Source: three-view drawing plus pictorial views. Frame: mm from the lowest corner of the part. Give positions to 0.01 mm unless a question says otherwise; leave off trailing zeros. Loops run counter-clockwise (first coordinate to the right, second up) from the corner with the lowest first, then second, coordinate; pieces in that order, holes last. Notation, with made-up numbers: (5.25, 73.5) -> (33.25, 73.5) arc R9 ccw to (33.25, 80.5) -> close; hole circle Ø6 at (51, 57). An arc over 180 degrees is marked (long way). Answer in a Markdown table with one row per item. Add a question column.
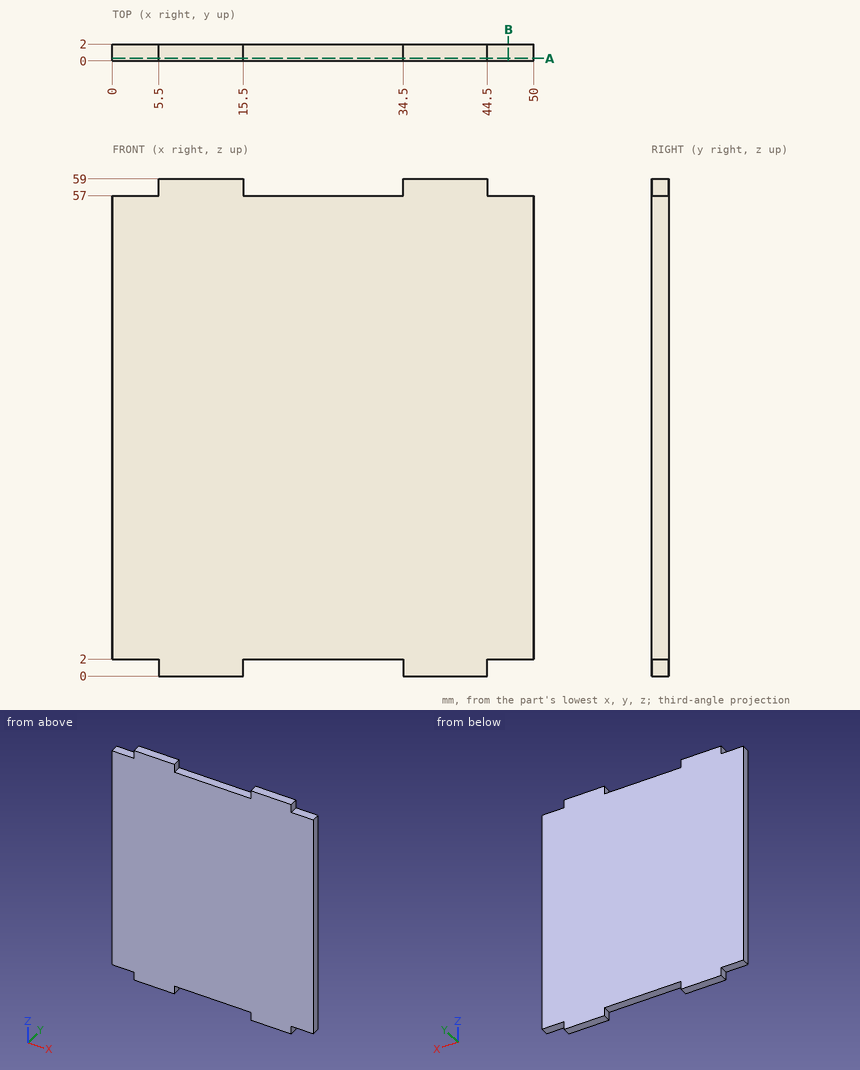
(1) Material intervals for line 1 along Z through (x, y) = (3, 1.25), sorted ascending. Write a range as from..to.
(2) Pin query (flat end, axial travel): pin 1 Ø5 at (x, z) = (39.5, 16.5) entering from -Y; pin 2 Ø1 at (x, y) = (47, 1) entering from -Z; pin 3 Ø0.6 at (y, z) = (0.5, 58) entering from -X; pin 4 Ø0.6 at (x, y) = (47.5, 1) entering from +Z. Return the tip coordinate at first contact, or that it passes through.
(3) Cut plane A-A on y = 0.3. Return the cut outline in (x, z), then the cut area to 3 significant figures.
(4) Cut plane B-B on x = 47. Return the cut outline in (y, z), then the cut area to 3 significant figures.
Answer list:
| question | item | result |
|---|---|---|
| 1 | line 1 | z = 2..57 |
| 2 | pin 1 | stops at y = 0 |
| 2 | pin 2 | stops at z = 2 |
| 2 | pin 3 | stops at x = 5.5 |
| 2 | pin 4 | stops at z = 57 |
| 3 | outline | (0, 2) -> (5.5, 2) -> (5.5, 0) -> (15.5, 0) -> (15.5, 2) -> (34.5, 2) -> (34.5, 0) -> (44.5, 0) -> (44.5, 2) -> (50, 2) -> (50, 57) -> (44.5, 57) -> (44.5, 59) -> (34.5, 59) -> (34.5, 57) -> (15.5, 57) -> (15.5, 59) -> (5.5, 59) -> (5.5, 57) -> (0, 57) -> close |
| 3 | area | 2,830 mm² |
| 4 | outline | (0, 2) -> (2, 2) -> (2, 57) -> (0, 57) -> close |
| 4 | area | 110 mm² |
